Design review of the part built by this model. Coordinates are the model's own, in mm. A direction names the side the tool comes from. Coordinates: 2 decimals unless noted, no trailing zeros. Loops run counter-clockwise (first coordinate to the right, second up) from the corner with the lowest first, then second, coordinate; pieces in that order, holes last.
Q1. For P1, Ø5, axis at x = 2, y = 10.5, coming from the +Z side; P2, Ø2, axis at y = 4.5, z = 22, coming from the -X side; P3, Ø6, axis at x = -10, z = 6, coming from the +Y side; P4, Ø12, axis at x = -11.5, z = 17.5, coming from the -Y side, all flat-tipped, find the tip position at first contact; note any pin that passes through.
Q2. Add section A-A on x = -1. Give the boundary of the cut face in (y, z), and give its area (3 significant figures).
Q3. Add section B-B on x = 12. Give the boundary of the cut face in (y, z), and give its area (3 significant figures).
Q4. Add section D-D on x = 25.1. Give the boundary of the cut face in (y, z).
Q5. Add section C-C on z = 8. Give the boundary of the cut face in (x, y).
Q6. Machinability: for faces 1 (the face through (-8, 6, 3.2)), 2 (the face through (0, 6, 24)), 3 (the face through (-8, 3.011, 5)), 4 (the face through (22.6, 6, 8)), which of the approach directions +Z, -Z, +X, -X, +Y, -Y give a long, thin tool a straight path to every point of the face, cutting with its end or side? Answer none if there is none.
Q7. Draft analysis for pull direction Z (two halves, no side actions). For faces 5 (the face through (7.26, 4.02, 27.78)), 6 (the face through (-4, 6, 15.6)), 7 (the face through (11, 6, 0)), 8 (the face through (-8, 6, 6.2)), state which applies: released by +Z, released by -Z, zero draft, split by the parting line, or undercut.
Q8. Wall thickness on probe 1 along Y at (x, z) = (25.1, 16.85); probe 2 along X at (y, z) = (2.5, 8.5); probe 3 along Z at (x, y) = (21, 9.75): over which ranges is each line inside the solid? List them lowest first.
```python
from build123d import *

# Parameters (mm, degrees)
ESQUISSE1_W             = 22.6
ESQUISSE1_H             = 12.3
BOSS_EXTRU_1_DEPTH      = 22.3
BOSS_EXTRU_2_DEPTH      = 5
BOSS_EXTRU_2_DEPTH_BACK = 27.6
ESQUISSE2_W             = 2.7
ESQUISSE2_H             = 12.3
ESQUISSE3_R             = 1.05
ENL_V_MAT_EXTRU_1_DEPTH = 5
BOSS_EXTRU_3_DEPTH      = 4
ESQUISSE5_R             = 2.4
BOSS_EXTRU_4_DEPTH      = 3
ESQUISSE6_W             = 3
ESQUISSE6_H             = 6.277768914
BOSS_EXTRU_5_DEPTH      = 16


with BuildPart() as part:
    # Esquisse1 → Boss.-Extru.1 (new body)
    with BuildSketch(Plane.XY):
        with Locations((11.3, 6.15)):
            Rectangle(ESQUISSE1_W, ESQUISSE1_H)
    extrude(amount=BOSS_EXTRU_1_DEPTH)

    # Esquisse2 → Boss.-Extru.2 (add, two sides: drawn at the far end of the back side and taken through both)
    with BuildSketch(Plane(origin=(22.6, 0, 0), x_dir=(0, 0, -1), z_dir=(1, 0, 0)).offset(-BOSS_EXTRU_2_DEPTH_BACK)):
        with Locations((-16.95, 6.15)):
            Rectangle(ESQUISSE2_W, ESQUISSE2_H)
    extrude(amount=BOSS_EXTRU_2_DEPTH + BOSS_EXTRU_2_DEPTH_BACK)

    # Esquisse3 → Enlèv. mat.-Extru.1 (cut)
    with BuildSketch(Plane.XY.offset(18.3)):
        with Locations((-2.5, 6.15)):
            Circle(ESQUISSE3_R)
        with Locations(Location((25.1, 6.15, 0), (0, 0, 90))):
            Circle(ESQUISSE3_R)
    extrude(amount=-ENL_V_MAT_EXTRU_1_DEPTH, mode=Mode.SUBTRACT)

    # Esquisse4 → Boss.-Extru.3 (add)
    with BuildSketch(Plane.XY.offset(22.3)):
        with BuildLine():
            ThreePointArc((11.304065041, 9.505311246), (0, 6.15), (11.304065041, 2.794688754))
            ThreePointArc((11.304065041, 2.794688754), (15.8, 6.15), (11.304065041, 9.505311246))
        make_face()
    extrude(amount=BOSS_EXTRU_3_DEPTH)

    # Esquisse5 → Boss.-Extru.4 (add)
    with BuildSketch(Plane.XY.offset(26.3)):
        with Locations((6.15, 6.15)):
            Circle(ESQUISSE5_R)
    extrude(amount=BOSS_EXTRU_4_DEPTH)

    # Esquisse6 → Boss.-Extru.5 (add)
    with BuildSketch(Plane.ZY):
        with Locations((4.7, 6.15)):
            Rectangle(ESQUISSE6_W, ESQUISSE6_H)
    extrude(amount=BOSS_EXTRU_5_DEPTH)


solid = part.part
```
Entries:
1. P1: stops at z = 26.3
1. P2: stops at x = 0
1. P3: stops at y = 9.29
1. P4: passes through
2. outline: (0, 15.6) - (12.3, 15.6) - (12.3, 18.3) - (0, 18.3) - close; (3.01, 3.2) - (9.29, 3.2) - (9.29, 6.2) - (3.01, 6.2) - close
2. area: 52.0 mm2
3. outline: (0, 0) - (12.3, 0) - (12.3, 22.3) - (9.64, 22.3) - (9.64, 26.3) - (2.66, 26.3) - (2.66, 22.3) - (0, 22.3) - close
3. area: 302 mm2
4. outline: (0, 15.6) - (5.1, 15.6) - (5.1, 18.3) - (0, 18.3) - close; (7.2, 15.6) - (12.3, 15.6) - (12.3, 18.3) - (7.2, 18.3) - close
5. outline: (0, 0) - (22.6, 0) - (22.6, 12.3) - (0, 12.3) - close
6. face 1: -Z, -X, +Y, -Y
6. face 2: +Z
6. face 3: -Z, -X, -Y
6. face 4: -Z, +X, +Y, -Y
7. face 5: zero draft
7. face 6: undercut
7. face 7: released by -Z
7. face 8: undercut
8. probe 1: y = 0 to 5.1, 7.2 to 12.3
8. probe 2: x = 0 to 22.6
8. probe 3: z = 0 to 22.3
